Input: dimensioned drawing with shaded views. Units: mm. Origin: part minimum x, y, z. A direction names the side the tool comes from. Coordinates: 2 decimals unless noted, no trailing zeros. Loops run counter-clockwise (first coordinate to the right, second up) from the corner with the lowest first, then second, coordinate; pieces in that order, holes last. Notation, with made-up numbers: (-25, 25) - (-18, 25) arc R17 cw to (-18, 38) - close; hole circle Ø11 at (-21.5, 74.5). An arc over 180 degrees is marked (long way). Use one line per item in the form item = value. Start each with the question number.
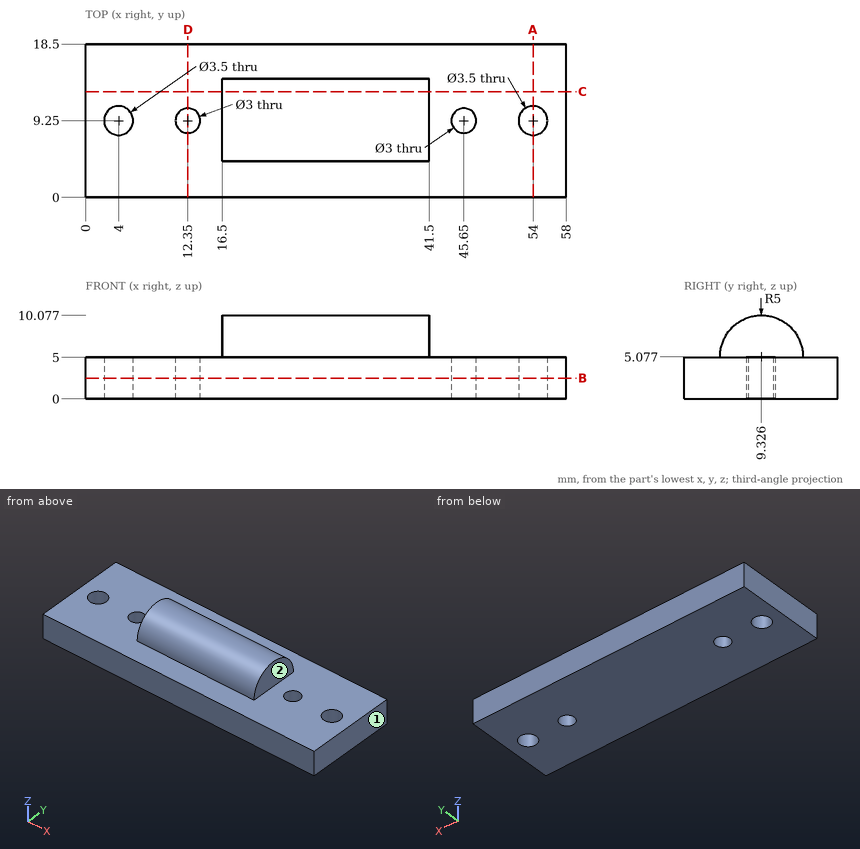
(1) Contact query for flat-ended pins moving along their axis: pin 1 (6 mm diameter, centred on y = 16, z = 8.5, fed in from +X); pin 2 (5.5 mm diameter, centred on y = 10.5, z = 8.5, fed in from -X); pin 3 (4 mm diameter, centred on x = 45.65, y = 9.25, fed in from +Z). Output: stop coordinate, or through.
(2) Material intervals for line 1 (Y direction, x = 4, z = 1.3); line 2 (Y direction, x = 45.65, z = 1); line 3 (X direction, y = 8.5, z = 2.5), sorted ascending.
(3) Cut plane A-A, the plane x = 54. Output: boundary loops of the cut face in (y, z), plus the area to 3 significant figures.
(4) Cut plane B-B, the plane z = 2.5. Output: boundary loops of the cut face in (x, y).
(5) Cut plane D-D, the plane x = 12.35. Output: boundary loops of the cut face in (y, z).
(6) Access query for the marked faces 1 and 2. Directions: +Z, -Z, +X, -X, +Y, -Y. A direction counts if a zero-diameter tool reaches every point of the face in a straight line with its end or side. Return the directions, or none.
(7) Cut plane C-C, the plane y = 12.75. Output: boundary loops of the cut face in (x, z).
Recorded:
q1.pin_1 = 41.5
q1.pin_2 = 16.5
q1.pin_3 = 5
q2.line_1 = 0 to 7.5, 11 to 18.5
q2.line_2 = 0 to 7.75, 10.75 to 18.5
q2.line_3 = 0 to 2.42, 5.58 to 11.05, 13.65 to 44.35, 46.95 to 52.42, 55.58 to 58
q3.outline = (0, 0) - (7.5, 0) - (7.5, 5) - (0, 5) - close; (11, 0) - (18.5, 0) - (18.5, 5) - (11, 5) - close
q3.area = 75.0 mm²
q4.outline = (0, 0) - (58, 0) - (58, 18.5) - (0, 18.5) - close; hole circle Ø3.5 at (4, 9.25); hole circle Ø3 at (12.35, 9.25); hole circle Ø3 at (45.65, 9.25); hole circle Ø3.5 at (54, 9.25)
q5.outline = (0, 0) - (7.75, 0) - (7.75, 5) - (0, 5) - close; (10.75, 0) - (18.5, 0) - (18.5, 5) - (10.75, 5) - close
q6.face_1 = +Z, -Z, +X, +Y, -Y
q6.face_2 = +Z, +X, +Y, -Y
q7.outline = (0, 0) - (58, 0) - (58, 5) - (41.5, 5) - (41.5, 8.72) - (16.5, 8.72) - (16.5, 5) - (0, 5) - close
